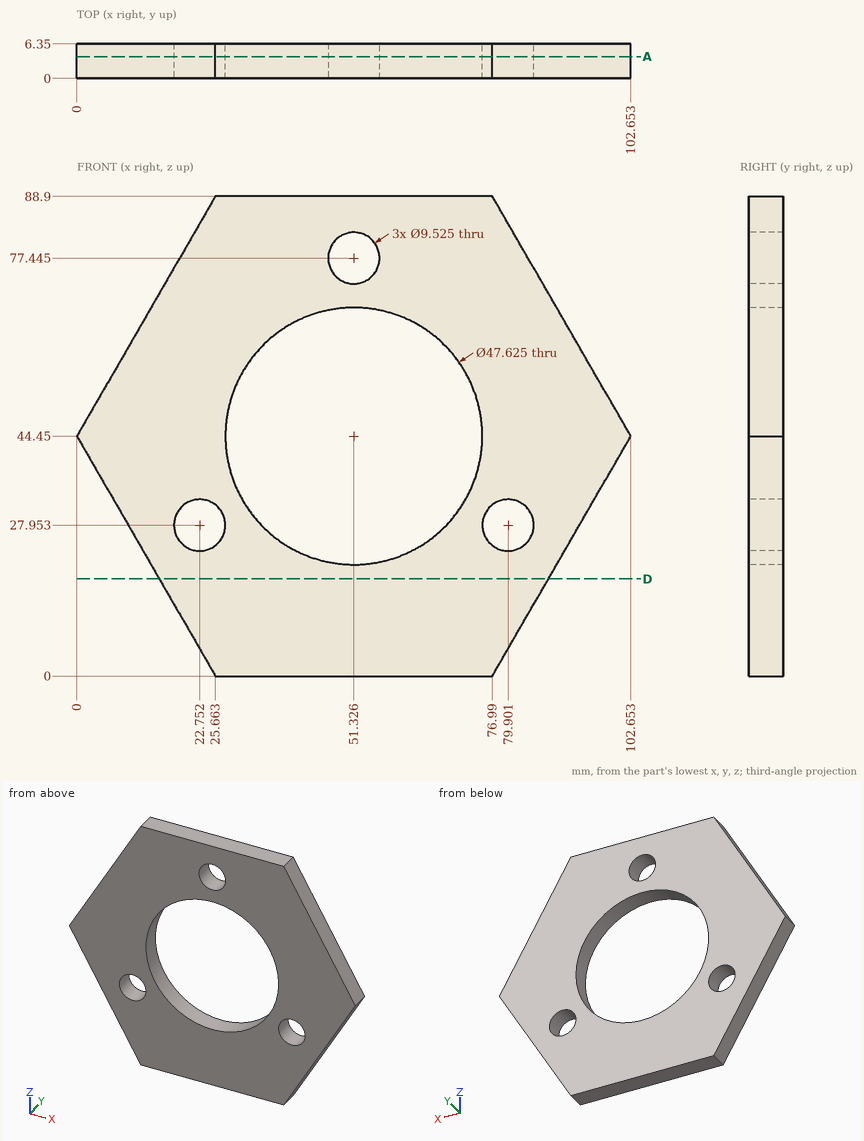
The figure shows three views and two pictorial views of one solid part (mm, origin at its lowest corner). Answer the questions. Give positions to 0.01 mm unless a question says otherwise; leave off trailing zeros. Loops run counter-clockwise (first coordinate to the right, second up) from the corner with the lowest first, then second, coordinate; pieces in that order, holes last. Notation, with made-up numbers: (57.25, 26.5) -> (100.25, 26.5) arc R18 ccw to (100.25, 35.5) -> close; hole circle Ø5 at (21.5, -6.5). An arc over 180 degrees is marked (long way). Put each result on its own line as item: value. Start each with the question number.
Item 1: The part is cut by section A-A (y = 4). State how many separate pieces and enclosed holes the cut face has, then the cut area to 3 significant figures.
Item 2: Find the intervals of material crossed by L1, parallel to X at y = 5.25, z = 30 (1 decimal); L2, parallel to X at y = 6.25, z = 57 (1 decimal); L3, parallel to Z at x = 33, y = 4 (1 decimal), in increasing order. Write a range as [from, to].
Item 3: The part is cut by section D-D (z = 18). Give the vertices of the cut face in (x, y).
Item 4: Each of these flat-tipped pins is pushed along its axis until it touches: P1, Ø1, axis at x = 27, z = 26, coming from the +Y side; P2, Ø1, axis at y = 2.5, z = 65.5, coming from the -X side (1 decimal); P3, Ø1.5, axis at y = 4.5, z = 33, coming from the -X side. Where does it stop, or does it pass through?
Answers below:
1. separate pieces: 1
1. enclosed holes: 4
1. area: 4,850 mm2
2. L1: [8.3, 18.5], [27.1, 32.4], [70.3, 75.6], [84.2, 94.3]
2. L2: [7.2, 31.1], [71.6, 95.4]
2. L3: [0, 29.2], [59.7, 88.9]
3. outline: (15.27, 0) -> (87.38, 0) -> (87.38, 6.35) -> (15.27, 6.35) -> close
4. P1: y = 6.35
4. P2: x = 11.9
4. P3: x = 6.18
